Source: CAD feature listing. Evaluate the final solid. Frame: model axes, mm. Face numbers are marked on the shaded views. A direction names the side the tool comes from. Give positions to 0.01 mm unless a question says otherwise; leave off trailing zeros. Order: outer loops, then holes, each group sorted by start corner. A loop starts at its lowest first (then second) coordinate and runs counter-clockwise, first axis right, second up.
1) Draft query along Y for the marked faces 1, 2, 3 and 4. Return one class per face: released by +Y, released by -Y, zero draft, split by the parting line, or undercut.
2) First-contact query: P1, Ø5, axis at y = 40.5, z = -58, coming from the -X side; P2, Ø1.8, axis at x = 40, z = -78, coming from the -Y side (1 decimal); P3, Ø5, axis at y = 35.5, z = -47.5, coming from the -X side; P4, Ø6.5, axis at y = 33.5, z = 3, coming from the +X side. Flat tips, straight axial feed; report the tip coordinate or a pass-through.
3) Access query for the marked faces 5, 6 and 7. Directions: +Z, -Z, +X, -X, +Y, -Y. A direction counts if a zero-diameter tool reaches every point of the face in a straight line with its end or side. Return the directions, or none.
4) Section A-A, the plane z = -36.5. Give the number of separate pieces and of enclosed holes in the cut face, plus the area to 3 significant figures.
5) Section D-D, the plane y = 44. Return loops of the section in (x, z).
6) Section C-C, the plane z = -16. Return loops of the section in (x, y).
7) Material intervals for line 1 (Z direction, x = 78, y = 16.2); line 2 (Y direction, x = 35, z = -18); line 3 (Y direction, x = 2.9, z = -35), sorted ascending.
8) Section B-B, the plane y = 37. Return loops of the section in (x, z).
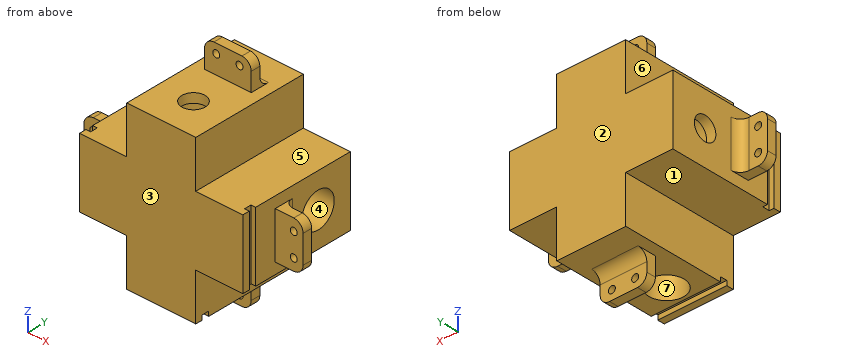
```python
from build123d import *

# Parameters (mm, degrees)
ESQUISSE1_W              = 70
ESQUISSE1_H              = 50
BOSS_EXTRU_1_DEPTH       = 70
ESQUISSE2_R              = 7.5
ENL_V_MAT_EXTRU_1_DEPTH  = 71
ESQUISSE3_R              = 7.5
ENL_V_MAT_EXTRU_2_DEPTH  = 71
ESQUISSE4_W              = 20.2
ESQUISSE4_H              = 20.2
ENL_V_MAT_EXTRU_3_DEPTH  = 51
ESQUISSE7_R              = 11.73674641
ESQUISSE7_R_2            = 5
BOSS_EXTRU_3_DEPTH       = 4
ESQUISSE8_R              = 12.196693844
ESQUISSE8_R_2            = 5
BOSS_EXTRU_4_DEPTH       = 4
ESQUISSE9_W              = 2
ESQUISSE9_H              = 3
ENL_V_MAT_EXTRU_4_DEPTH  = 50.8
ESQUISSE10_W             = 2
ESQUISSE10_H             = 3
ENL_V_MAT_EXTRU_5_DEPTH  = 50.8
ESQUISSE11_W             = 2
ESQUISSE11_H             = 3
ENL_V_MAT_EXTRU_6_DEPTH  = 50.8
ESQUISSE12_W             = 20
ESQUISSE12_H             = 4
BOSS_EXTRU_5_DEPTH       = 12
ESQUISSE13_R             = 1.5
ENL_V_MAT_EXTRU_7_DEPTH  = 36
CONG_1_R                 = 4
ESQUISSE14_W             = 20
ESQUISSE14_H             = 4
BOSS_EXTRU_6_DEPTH       = 12
ESQUISSE15_R             = 1.5
ENL_V_MAT_EXTRU_8_DEPTH  = 36
CONG_3_R                 = 4
ESQUISSE16_W             = 20
ESQUISSE16_H             = 4
BOSS_EXTRU_7_DEPTH       = 12
ESQUISSE17_R             = 1.5
ENL_V_MAT_EXTRU_9_DEPTH  = 20
CONG_4_R                 = 4
ESQUISSE18_W             = 20
ESQUISSE18_H             = 4
BOSS_EXTRU_8_DEPTH       = 12
ESQUISSE19_R             = 1.5
ENL_V_MAT_EXTRU_10_DEPTH = 20
CONG_5_R                 = 4
CONG_6_R                 = 4


with BuildPart() as part:
    # Esquisse1 → Boss.-Extru.1 (new body)
    with BuildSketch(Plane(origin=(0, 0, 0), x_dir=(0, 0, -1), z_dir=(1, 0, 0))):
        with Locations((35, 25)):
            Rectangle(ESQUISSE1_W, ESQUISSE1_H)
    extrude(amount=BOSS_EXTRU_1_DEPTH)

    # Esquisse2 → Enlèv. mat.-Extru.1 (cut, through all)
    with BuildSketch(Plane.XY):
        with Locations((35, 15)):
            Circle(ESQUISSE2_R)
    extrude(amount=-ENL_V_MAT_EXTRU_1_DEPTH, mode=Mode.SUBTRACT)

    # Esquisse3 → Enlèv. mat.-Extru.2 (cut, through all)
    with BuildSketch(Plane.ZY):
        with Locations((-35, 35)):
            Circle(ESQUISSE3_R)
    extrude(amount=-ENL_V_MAT_EXTRU_2_DEPTH, mode=Mode.SUBTRACT)

    # Esquisse4 → Enlèv. mat.-Extru.3 (cut, through all)
    with BuildSketch(Plane.XZ):
        with Locations((10.1, -59.9)):
            Rectangle(ESQUISSE4_W, ESQUISSE4_H)
        with Locations((10.1, -10.1)):
            Rectangle(ESQUISSE4_W, ESQUISSE4_H)
        with Locations((59.9, -10.1)):
            Rectangle(ESQUISSE4_W, ESQUISSE4_H)
        with Locations((59.9, -59.9)):
            Rectangle(ESQUISSE4_W, ESQUISSE4_H)
    extrude(amount=-ENL_V_MAT_EXTRU_3_DEPTH, mode=Mode.SUBTRACT)

    # Esquisse7 → Boss.-Extru.3 (add)
    with BuildSketch(Plane.XY):
        with Locations((35, 15)):
            Circle(ESQUISSE7_R)
        with Locations((35, 15)):
            Circle(ESQUISSE7_R_2, mode=Mode.SUBTRACT)
    extrude(amount=-BOSS_EXTRU_3_DEPTH)

    # Esquisse8 → Boss.-Extru.4 (add)
    with BuildSketch(Plane.ZY):
        with Locations((-35, 35)):
            Circle(ESQUISSE8_R)
        with Locations((-35, 35)):
            Circle(ESQUISSE8_R_2, mode=Mode.SUBTRACT)
    extrude(amount=-BOSS_EXTRU_4_DEPTH)

    # Esquisse9 → Enlèv. mat.-Extru.4 (cut, through all)
    with BuildSketch(Plane.ZY.offset(-20.2)):
        with Locations((-69, 4.5)):
            Rectangle(ESQUISSE9_W, ESQUISSE9_H)
    extrude(amount=-ENL_V_MAT_EXTRU_4_DEPTH, mode=Mode.SUBTRACT)

    # Esquisse10 → Enlèv. mat.-Extru.5 (cut, through all)
    with BuildSketch(Plane(origin=(0, 0, -49.8), x_dir=(-1, 0, 0), z_dir=(0, 0, -1))):
        with Locations((-1, 4.5)):
            Rectangle(ESQUISSE10_W, ESQUISSE10_H)
    extrude(amount=-ENL_V_MAT_EXTRU_5_DEPTH, mode=Mode.SUBTRACT)

    # Esquisse11 → Enlèv. mat.-Extru.6 (cut, through all)
    with BuildSketch(Plane(origin=(0, 0, -49.8), x_dir=(-1, 0, 0), z_dir=(0, 0, -1))):
        with Locations((-69, 4.5)):
            Rectangle(ESQUISSE11_W, ESQUISSE11_H)
    extrude(amount=-ENL_V_MAT_EXTRU_6_DEPTH, mode=Mode.SUBTRACT)

    # Esquisse12 → Boss.-Extru.5 (add)
    with BuildSketch(Plane.ZY):
        with Locations((-35, 17)):
            Rectangle(ESQUISSE12_W, ESQUISSE12_H)
    extrude(amount=BOSS_EXTRU_5_DEPTH)

    # Esquisse13 → Enlèv. mat.-Extru.7 (cut, through all)
    with BuildSketch(Plane.XZ.offset(-15)):
        with Locations(Location((-8, -30, 0), (0, 0, 270))):  # turned: the seam where the file's is
            Circle(ESQUISSE13_R)
        with Locations(Location((-8, -40, 0), (0, 0, 270))):  # turned: the seam where the file's is
            Circle(ESQUISSE13_R)
    extrude(amount=-ENL_V_MAT_EXTRU_7_DEPTH, mode=Mode.SUBTRACT)

    # Congé1
    cong_1_edges = [part.edges().sort_by_distance(p)[0] for p in [
        (-12, 17, -25),
        (-12, 17, -45),
    ]]
    fillet(cong_1_edges, radius=CONG_1_R)

    # Esquisse14 → Boss.-Extru.6 (add)
    with BuildSketch(Plane(origin=(70, 0, 0), x_dir=(0, 0, -1), z_dir=(1, 0, 0))):
        with Locations((35, 17)):
            Rectangle(ESQUISSE14_W, ESQUISSE14_H)
    extrude(amount=BOSS_EXTRU_6_DEPTH)

    # Esquisse15 → Enlèv. mat.-Extru.8 (cut, through all)
    with BuildSketch(Plane.XZ.offset(-15)):
        with Locations(Location((78, -40, 0), (0, 0, 270))):  # turned: the seam where the file's is
            Circle(ESQUISSE15_R)
        with Locations(Location((78, -30, 0), (0, 0, 270))):  # turned: the seam where the file's is
            Circle(ESQUISSE15_R)
    extrude(amount=-ENL_V_MAT_EXTRU_8_DEPTH, mode=Mode.SUBTRACT)

    # Congé3
    cong_3_edges = [part.edges().sort_by_distance(p)[0] for p in [
        (82, 17, -45),
        (82, 17, -25),
    ]]
    fillet(cong_3_edges, radius=CONG_3_R)

    # Esquisse16 → Boss.-Extru.7 (add)
    with BuildSketch(Plane.XY):
        with Locations((35, 33)):
            Rectangle(ESQUISSE16_W, ESQUISSE16_H)
    extrude(amount=BOSS_EXTRU_7_DEPTH)

    # Esquisse17 → Enlèv. mat.-Extru.9 (cut, through all)
    with BuildSketch(Plane.XZ.offset(-31)):
        with Locations((40, 8)):
            Circle(ESQUISSE17_R)
        with Locations((30, 8)):
            Circle(ESQUISSE17_R)
    extrude(amount=-ENL_V_MAT_EXTRU_9_DEPTH, mode=Mode.SUBTRACT)

    # Congé4
    cong_4_edges = [part.edges().sort_by_distance(p)[0] for p in [
        (45, 33, 12),
        (25, 33, 12),
    ]]
    fillet(cong_4_edges, radius=CONG_4_R)

    # Esquisse18 → Boss.-Extru.8 (add)
    with BuildSketch(Plane(origin=(0, 0, -70), x_dir=(-1, 0, 0), z_dir=(0, 0, -1))):
        with Locations((-35, 33)):
            Rectangle(ESQUISSE18_W, ESQUISSE18_H)
    extrude(amount=BOSS_EXTRU_8_DEPTH)

    # Esquisse19 → Enlèv. mat.-Extru.10 (cut, through all)
    with BuildSketch(Plane.XZ.offset(-31)):
        with Locations((30, -78)):
            Circle(ESQUISSE19_R)
        with Locations((40, -78)):
            Circle(ESQUISSE19_R)
    extrude(amount=-ENL_V_MAT_EXTRU_10_DEPTH, mode=Mode.SUBTRACT)

    # Congé5
    cong_5_edges = [part.edges().sort_by_distance(p)[0] for p in [
        (25, 33, -82),
        (45, 33, -82),
    ]]
    fillet(cong_5_edges, radius=CONG_5_R)

    # Congé6
    cong_6_edges = [part.edges().sort_by_distance(p)[0] for p in [
        (0, 19, -35),
        (70, 19, -35),
        (35, 35, 0),
        (35, 35, -70),
    ]]
    fillet(cong_6_edges, radius=CONG_6_R)


solid = part.part
```
From the geometry:
1. face 1: zero draft
1. face 2: released by +Y
1. face 3: released by -Y
1. face 4: undercut
2. P1: stops at x = 20.2
2. P2: passes through
2. P3: stops at x = 0
2. P4: stops at x = 49.8
3. face 5: +Z, +X, +Y, -Y
3. face 6: +Z, -X, +Y, -Y
3. face 7: -Z
4. separate pieces: 2
4. enclosed holes: 1
4. area: 2,410 mm2
5. outline: (0, -49.8) - (20.2, -49.8) - (20.2, -70) - (49.8, -70) - (49.8, -49.8) - (70, -49.8) - (70, -20.2) - (49.8, -20.2) - (49.8, 0) - (20.2, 0) - (20.2, -20.2) - (0, -20.2) - close
6. outline: (20.2, 0) - (49.8, 0) - (49.8, 50) - (20.2, 50) - close; hole circle Ø15 at (35, 15)
7. line 1: z = -45 to -41.5, -38.5 to -31.5, -28.5 to -25
7. line 2: y = 0 to 7.5, 22.5 to 50
7. line 3: y = 0 to 30, 40 to 50
8. outline: (0, -49.8) - (20.2, -49.8) - (20.2, -70) - (25, -70) - (25, -70.54) - (45, -70.54) - (45, -70) - (49.8, -70) - (49.8, -49.8) - (70, -49.8) - (70, -42.23) - (4, -42.23) - (4, -39.58) - (0, -39.58) - close; (0, -30.42) - (4, -30.42) - (4, -27.77) - (70, -27.77) - (70, -20.2) - (49.8, -20.2) - (49.8, 0) - (45, 0) - (45, 0.54) - (25, 0.54) - (25, 0) - (20.2, 0) - (20.2, -20.2) - (0, -20.2) - close
